Build history of the part. All positions in model axes, mm. Face numbers are marked on the shaded views. A direction names the side the tool comes from. Give positions to 0.01 mm unless a question says otherwise; leave off trailing zeros. Order: outer loops, then holes, each group sorted by start corner. A loop starts at its lowest first (then second) coordinate and runs counter-clockwise, first axis right, second up. Notation, with made-up numbers: M 25.5,54.5 L 84.5,54.5 A21 ccw 84.5,64.5 Z; hole C 3,41.25 d11. An arc over 180 degrees is marked long. One line per item, written item: value. Start each with the question number.
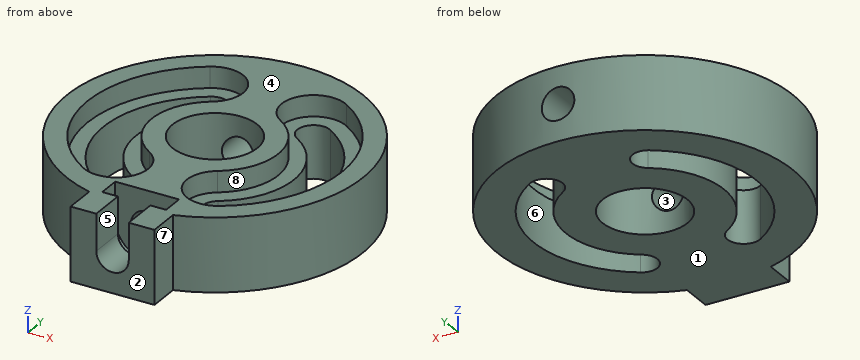
from build123d import *

# Parameters (mm, degrees)
SKETCH_R        = 4.05
EXTRUDE_DEPTH   = 7
SKETCH001_R     = 1.55
POCKET_DEPTH    = 30.723859
POCKET001_DEPTH = 3.5
POCKET002_DEPTH = 2.1
POCKET003_DEPTH = 2


with BuildPart() as part:
    # Sketch → Extrude (new body)
    with BuildSketch(Plane.XY):
        with BuildLine():
            ThreePointArc((4, -13.572859), (0, 14.15), (-4, -13.572859))
            Line((-4, -13.572859), (-4, -16.572859))
            Line((-4, -16.572859), (4, -16.572859))
            Line((4, -16.572859), (4, -13.572859))
        make_face()
        Circle(SKETCH_R, mode=Mode.SUBTRACT)
        with BuildLine():
            ThreePointArc((-4.056612, 6.367605), (-7.55, 0), (-4.056612, -6.367605))
            ThreePointArc((-5.722241, -8.982119), (-3.58217, -8.507677), (-4.056612, -6.367605))
            ThreePointArc((-5.722241, 8.982119), (-10.65, 0), (-5.722241, -8.982119))
            ThreePointArc((-4.056612, 6.367605), (-3.58217, 8.507677), (-5.722241, 8.982119))
        make_face(mode=Mode.SUBTRACT)
        with BuildLine():
            ThreePointArc((4.056612, -6.367605), (7.55, 0), (4.056612, 6.367605))
            ThreePointArc((5.722241, 8.982119), (3.58217, 8.507677), (4.056612, 6.367605))
            ThreePointArc((5.722241, -8.982119), (10.65, 0), (5.722241, 8.982119))
            ThreePointArc((4.056612, -6.367605), (3.58217, -8.507677), (5.722241, -8.982119))
        make_face(mode=Mode.SUBTRACT)
    extrude(amount=EXTRUDE_DEPTH)

    # Sketch001 → Pocket (cut, through all)
    with BuildSketch(Plane.XZ.offset(16.572859)):
        with Locations((0, 3.5)):
            Circle(SKETCH001_R)
    extrude(amount=-POCKET_DEPTH, mode=Mode.SUBTRACT)

    # Sketch002 → Pocket001 (cut)
    with BuildSketch(Plane.XY.offset(7)):
        Polygon((-3.049999, -10.972859), (-3.049999, -13.072859), (-1.549999, -13.072859), (-1.549999, -16.572859), (1.550001, -16.572859), (1.550001, -13.072859), (3.050001, -13.072859), (3.050001, -10.972859), align=None)
    extrude(amount=-POCKET001_DEPTH, mode=Mode.SUBTRACT)

    # Sketch003 → Pocket002 (cut)
    with BuildSketch(Plane.XZ.offset(10.972859)):
        with BuildLine():
            ThreePointArc((-3.050001, 3.5), (0, 0.449999), (3.050001, 3.5))
            Line((-3.050001, 3.5), (3.050001, 3.5))
        make_face()
    extrude(amount=POCKET002_DEPTH, mode=Mode.SUBTRACT)

    # Sketch004 → Pocket003 (cut)
    with BuildSketch(Plane.XY.offset(7)):
        with BuildLine():
            ThreePointArc((-3.250663, 5.102518), (-2.317083, 9.313626), (-6.52819, 10.247206))
            ThreePointArc((-6.52819, 10.247206), (-12.15, 0), (-6.52819, -10.247206))
            ThreePointArc((-6.52819, -10.247206), (-2.317083, -9.313626), (-3.250663, -5.102518))
            ThreePointArc((-3.250663, 5.102518), (-6.05, 0), (-3.250663, -5.102518))
        make_face()
        with BuildLine():
            ThreePointArc((6.52819, 10.247206), (2.317083, 9.313626), (3.250663, 5.102518))
            ThreePointArc((3.250663, -5.102518), (6.05, 0), (3.250663, 5.102518))
            ThreePointArc((3.250663, -5.102518), (2.317083, -9.313626), (6.52819, -10.247206))
            ThreePointArc((6.52819, -10.247206), (12.15, 0), (6.52819, 10.247206))
        make_face()
    extrude(amount=-POCKET003_DEPTH, mode=Mode.SUBTRACT)


solid = part.part
1) Slice it at B-B (z = 4). List the corners of the cut face in (x, y).
2) Pull direction Z, two halves, no side cores. Call the marked faces 1, 2, 3 and 4: pulls with the +Z half, pulls with the -Z half, needs draft (parallel to the pull), parting line crosses it, or undercut.
3) Tool access for the marked faces 5, 6, 7 and 8: list every direction of +Z, -Z, +X, -X, +Y, -Y with a clear straight run to the whole face (end or side of a thin tool).
4) Drill centre lines: line 1 (Z direction, x = 0, y = -8.5); line 2 (X direction, y = 3.5, z = 0.5); line 3 (Y direction, x = -1, z = 1.5). Where is each one in solid material? Low to high.
5) Slice it at A-A (x = 0). List the corners of the cut face in (y, z).
6) Drop flat-ended pins along their axis: P1, Ø0.9, axis at y = -15.5, z = 4, coming from the +X side; P2, Ø1.7, axis at y = -12.5, z = 6, coming from the -X side; P3, Ø1, axis at x = 9, y = -9, coming from the -Z side; P4, Ø3, axis at y = -15.5, z = 5, coming from the -X side. Give the stop position or say it passes through.
7) Slice it at D-D (z = 6). List the corners of the cut face in (x, y).
8) Slice it at C-C (y = 1). List the corners of the cut face in (x, z).
Results list:
1. outline: M -4,-16.57 L -1.55,-16.57 L -1.55,-13.07 L -3.05,-13.07 L -3.05,-10.97 L -1.47,-10.97 L -1.47,-3.77 A4.05 cw -1.47,3.77 L -1.47,14.07 A14.15 ccw -4,-13.57 Z; M 1.47,-10.97 L 3.05,-10.97 L 3.05,-13.07 L 1.55,-13.07 L 1.55,-16.57 L 4,-16.57 L 4,-13.57 A14.15 ccw 1.47,14.07 L 1.47,3.77 A4.05 cw 1.47,-3.77 Z; hole M -5.72,-8.98 A1.55 ccw -4.06,-6.37 A7.55 cw -4.06,6.37 A1.55 ccw -5.72,8.98 A10.65 ccw Z; hole M 4.06,-6.37 A1.55 ccw 5.72,-8.98 A10.65 ccw 5.72,8.98 A1.55 ccw 4.06,6.37 A7.55 cw Z
2. face 1: pulls with the -Z half
2. face 2: needs draft
2. face 3: undercut
2. face 4: pulls with the +Z half
3. face 5: +Z, -Y
3. face 6: +Z, -Z
3. face 7: +Z, -Z, +X, -Y
3. face 8: +Z
4. line 1: z = 0 to 1.95, 5.05 to 7
4. line 2: x = -13.71 to -10.06, -6.69 to -2.04, 2.04 to 6.69, 10.06 to 13.71
4. line 3: y = -16.57 to -13.07, -10.97 to -3.92, 3.92 to 14.11
5. outline: M -16.57,0 L -4.05,0 L -4.05,1.95 L -10.97,1.95 L -10.97,0.45 L -13.07,0.45 L -13.07,1.95 L -16.57,1.95 Z; M -10.97,5.05 L -4.05,5.05 L -4.05,7 L -10.97,7 Z; M 4.05,0 L 14.15,0 L 14.15,1.95 L 4.05,1.95 Z; M 4.05,5.05 L 14.15,5.05 L 14.15,7 L 4.05,7 Z
6. P1: stops at x = 4
6. P2: stops at x = -8.03
6. P3: stops at z = 0
6. P4: stops at x = -4
7. outline: M -4,-16.57 L -1.55,-16.57 L -1.55,-13.07 L -3.05,-13.07 L -3.05,-10.97 L 3.05,-10.97 L 3.05,-13.07 L 1.55,-13.07 L 1.55,-16.57 L 4,-16.57 L 4,-13.57 A14.15 ccw long -4,-13.57 Z; hole M -6.53,-10.25 A3.05 ccw -3.25,-5.1 A6.05 cw -3.25,5.1 A3.05 ccw -6.53,10.25 A12.15 ccw Z; hole C 0,0 d8.1; hole M 3.25,-5.1 A3.05 ccw 6.53,-10.25 A12.15 ccw 6.53,10.25 A3.05 ccw 3.25,5.1 A6.05 cw Z
8. outline: M -14.11,0 L -10.6,0 L -10.6,5 L -12.11,5 L -12.11,7 L -14.11,7 Z; M -7.48,0 L -3.92,0 L -3.92,7 L -5.97,7 L -5.97,5 L -7.48,5 Z; M 3.92,0 L 7.48,0 L 7.48,5 L 5.97,5 L 5.97,7 L 3.92,7 Z; M 10.6,0 L 14.11,0 L 14.11,7 L 12.11,7 L 12.11,5 L 10.6,5 Z
